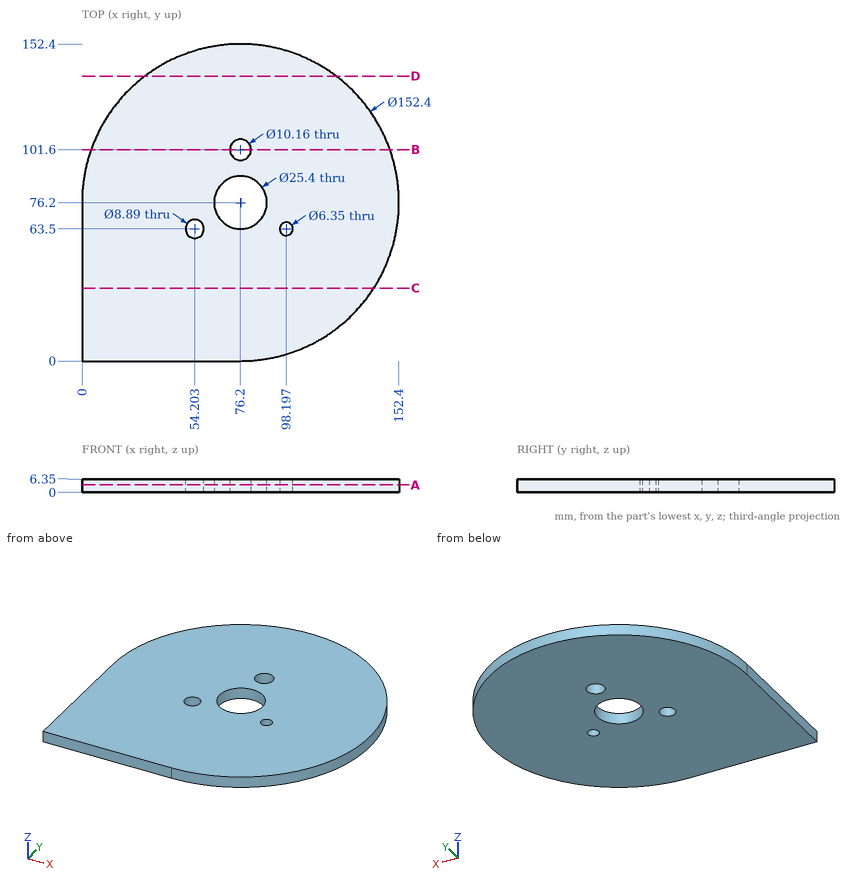
For this review, use the dimensioned drawing (mm, ordinates from the lowest corner) and the shaded views. Coordinates: 2 decimals unless noted, no trailing zeros. Write each loop counter-clockwise with the first axis right and the second up, starting at its lowest first coordinate (ties: lowest second). Pieces come first, ordered by that corner, then holes. Notation, with made-up numbers: (82.25, -24) - (128.25, -24) arc R23 cw to (128.25, 7) - close; hole circle Ø7 at (-29.75, 6.25). An arc over 180 degrees is marked (long way). One line per item, written item: value.
1) Add section D-D (y = 137). State the section outline as (x, z) points, plus the area to 3 significant figures.
Answer sheet:
outline: (30.27, 0) - (122.13, 0) - (122.13, 6.35) - (30.27, 6.35) - close
area: 583 mm2
2) Add section A-A (z = 3.5). State the section outline as (x, y) points (3 decimals), plus the area to 3 significant figures.
Answer sheet:
outline: (0, 0) - (76.2, 0) arc R76.2 ccw (long way) to (0, 76.2) - close; hole circle Ø8.89 at (54.203, 63.5); hole circle Ø25.4 at (76.2, 76.2); hole circle Ø10.16 at (76.2, 101.6); hole circle Ø6.35 at (98.197, 63.5)
area: 18,800 mm2
3) Insertion check: pin 1 (5 mm diameter, centred on x = 98.2, y = 63.5, fed in from +Z). The pin has a flat end and moves straight along its axis. Give the tip position at first contact, or say it passes through.
Answer sheet:
pin 1: passes through
4) To check wall thickness, follow probe 1 along Y at (x, z) = (76.2, 3); probe 2 along Y at (x, z) = (74, 4.5); probe 3 along X at (y, z) = (74.5, 3). State the ranges of each line that lie inside material, in increasing order.
Answer sheet:
probe 1: y = 0 to 63.5, 88.9 to 96.52, 106.68 to 152.4
probe 2: y = 0 to 63.69, 88.71 to 97.02, 106.18 to 152.37
probe 3: x = 0 to 63.61, 88.79 to 152.38
5) Add section C-C (y = 35). State the section outline as (x, z) points.
Answer sheet:
outline: (0, 0) - (140.3, 0) - (140.3, 6.35) - (0, 6.35) - close
6) Add section B-B (y = 101.6). State the section outline as (x, z) points, plus the area to 3 significant figures.
Answer sheet:
outline: (4.36, 0) - (71.12, 0) - (71.12, 6.35) - (4.36, 6.35) - close; (81.28, 0) - (148.04, 0) - (148.04, 6.35) - (81.28, 6.35) - close
area: 848 mm2
